For this review, take the finished solid that the model builds, in its own axes (mm). Face numbers are marked on the shaded views. A direction names the side the tool comes from. Give positions to 0.01 mm unless a question says otherwise; leave off trailing zeros. Write each loop counter-clockwise with the first axis right and the second up, starting at its lowest first coordinate (ties: lowest second). Pieces come first, ordered by that corner, then holes. Notation, with made-up numbers: M 17.25,-11.75 L 43.25,-11.75 A10 cw 43.25,-5.75 Z; hole C 64.5,-21.75 d8. An arc over 180 degrees is marked long. Use one line per item in the form item = value. Start each with the question number.
Q1. Clearance check with flat-ended pins moving along their axes: pin 1 Ø12 at (x, z) = (12, -5) entering from +Y; pin 2 Ø2 at (x, y) = (4, 32.5) entering from -Z; pin 3 Ø21.5 at (x, y) = (-8.5, 23) entering from +Z. State where each tip first meets the part, or that it passes through.
Q2. Consider section C-C on y = 21.5. Write out the cut boundary in (x, z), and give its area (3 significant figures).
Q3. Consider section D-D on z = -31. Write out the cut boundary in (x, y).
Q4. Consider section B-B on x = -15.5. Write out the cut boundary in (y, z).
Q5. Tool access review of the marked faces 1, 2 and 3: name each direction out of +Z, -Z, +X, -X, +Y, -Y from which nothing blocks a thin tool from reaching the whole face with its end or side.
Q6. For probe 1 along X at (y, z) = (-1, 31); probe 2 along Z at (x, y) = (-11, -1); probe 3 along Y at (x, z) = (11, 27), list the stretches that pass through material, from the lowest coordinate up. Write a range as [from, to].
Q7. Consider section A-A on y = 6. Write out the cut boundary in (x, z).
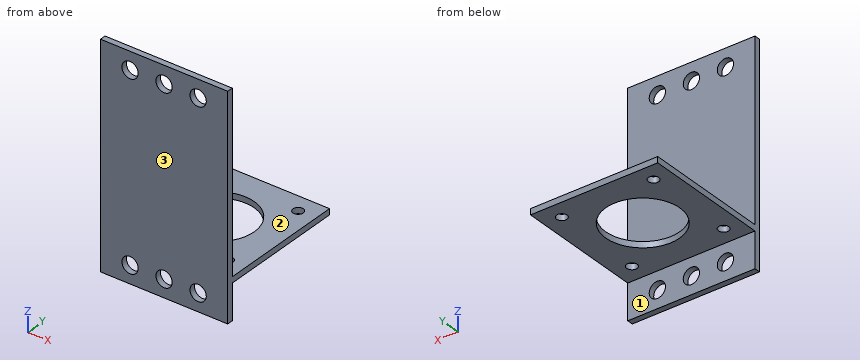
```python
from build123d import *

# Parameters (mm, degrees)
SKETCH1_W           = 43
SKETCH1_H           = 2
BOSS_EXTRUDE1_DEPTH = 43
SKETCH1_3_W         = 43
SKETCH1_3_H         = 74
BOSS_EXTRUDE2_DEPTH = 2
CUT_EXTRUDE1_REACH  = 78.885
SKETCH2_R           = 12.5
SKETCH2_R_2         = 1.75
CUT_EXTRUDE2_REACH  = 62.665
SKETCH1_4_R         = 2.75
LPATTERN1_COUNT     = 2
LPATTERN1_PITCH     = 11.5
LPATTERN1_COL_COUNT = 2
LPATTERN1_COL_PITCH = 11.5


with BuildPart() as part:
    # Sketch1 → Boss-Extrude1 (new body)
    with BuildSketch(Plane(origin=(0, 0, 0), x_dir=(1, 0, 0), z_dir=(0, 1, 0))):
        with Locations((0, 24)):
            Rectangle(SKETCH1_W, SKETCH1_H)
    extrude(amount=BOSS_EXTRUDE1_DEPTH)

    # Sketch1_3 → Boss-Extrude2 (add)
    with BuildSketch(Plane(origin=(0, 0, 0), x_dir=(1, 0, 0), z_dir=(0, 1, 0))):
        Rectangle(SKETCH1_3_W, SKETCH1_3_H)
    extrude(amount=-BOSS_EXTRUDE2_DEPTH)

    # Sketch2 → Cut-Extrude1 (cut, up to next)
    with BuildSketch(Plane.XY.offset(-23), mode=Mode.PRIVATE) as cut_extrude1_sk1:
        with Locations((0, 21.5)):
            Circle(SKETCH2_R)
    cut_extrude1_tool1 = extrude(cut_extrude1_sk1.sketch, amount=-CUT_EXTRUDE1_REACH, mode=Mode.PRIVATE) & part.part
    # Sketch2 → Cut-Extrude1 (cut, up to next)
    with BuildSketch(Plane.XY.offset(-23), mode=Mode.PRIVATE) as cut_extrude1_sk2:
        with Locations((-15.5, 37)):
            Circle(SKETCH2_R_2)
    cut_extrude1_tool2 = extrude(cut_extrude1_sk2.sketch, amount=-CUT_EXTRUDE1_REACH, mode=Mode.PRIVATE) & part.part
    # Sketch2 → Cut-Extrude1 (cut, up to next)
    with BuildSketch(Plane.XY.offset(-23), mode=Mode.PRIVATE) as cut_extrude1_sk3:
        with Locations((15.5, 37)):
            Circle(SKETCH2_R_2)
    cut_extrude1_tool3 = extrude(cut_extrude1_sk3.sketch, amount=-CUT_EXTRUDE1_REACH, mode=Mode.PRIVATE) & part.part
    # Sketch2 → Cut-Extrude1 (cut, up to next)
    with BuildSketch(Plane.XY.offset(-23), mode=Mode.PRIVATE) as cut_extrude1_sk4:
        with Locations((15.5, 6)):
            Circle(SKETCH2_R_2)
    cut_extrude1_tool4 = extrude(cut_extrude1_sk4.sketch, amount=-CUT_EXTRUDE1_REACH, mode=Mode.PRIVATE) & part.part
    # Sketch2 → Cut-Extrude1 (cut, up to next)
    with BuildSketch(Plane.XY.offset(-23), mode=Mode.PRIVATE) as cut_extrude1_sk5:
        with Locations((-15.5, 6)):
            Circle(SKETCH2_R_2)
    cut_extrude1_tool5 = extrude(cut_extrude1_sk5.sketch, amount=-CUT_EXTRUDE1_REACH, mode=Mode.PRIVATE) & part.part
    add(cut_extrude1_tool1.solids().sort_by_distance((0, 21.5, -23))[0], mode=Mode.SUBTRACT)
    add(cut_extrude1_tool2.solids().sort_by_distance((-15.5, 37, -23))[0], mode=Mode.SUBTRACT)
    add(cut_extrude1_tool3.solids().sort_by_distance((15.5, 37, -23))[0], mode=Mode.SUBTRACT)
    add(cut_extrude1_tool4.solids().sort_by_distance((15.5, 6, -23))[0], mode=Mode.SUBTRACT)
    add(cut_extrude1_tool5.solids().sort_by_distance((-15.5, 6, -23))[0], mode=Mode.SUBTRACT)

    # Sketch1_4 → Cut-Extrude2 (cut, up to next)
    with BuildSketch(Plane(origin=(0, 0, 0), x_dir=(1, 0, 0), z_dir=(0, 1, 0)), mode=Mode.PRIVATE) as cut_extrude2_sk1:
        with Locations(Location((0, 31, 0), (0, 0, 270))):
            Circle(SKETCH1_4_R)
    cut_extrude2_tool1 = extrude(cut_extrude2_sk1.sketch, amount=-CUT_EXTRUDE2_REACH, mode=Mode.PRIVATE) & part.part
    # Sketch1_4 → Cut-Extrude2 (cut, up to next)
    with BuildSketch(Plane(origin=(0, 0, 0), x_dir=(1, 0, 0), z_dir=(0, 1, 0)), mode=Mode.PRIVATE) as cut_extrude2_sk2:
        with Locations(Location((0, -31, 0), (0, 0, 270))):
            Circle(SKETCH1_4_R)
    cut_extrude2_tool2 = extrude(cut_extrude2_sk2.sketch, amount=-CUT_EXTRUDE2_REACH, mode=Mode.PRIVATE) & part.part
    cut_extrude2_1 = cut_extrude2_tool1.solids().sort_by_distance((0, 0, -31))[0]
    add(cut_extrude2_1, mode=Mode.SUBTRACT)
    cut_extrude2_2 = cut_extrude2_tool2.solids().sort_by_distance((0, 0, 31))[0]
    add(cut_extrude2_2, mode=Mode.SUBTRACT)
    cut_extrude2 = cut_extrude2_1 + cut_extrude2_2  # Cut-Extrude2 as one shape, for the pattern or mirror that repeats it

    # LPattern1: Cut-Extrude2 ×2
    with Locations(*[(i * LPATTERN1_PITCH, 0, 0) for i in range(1, LPATTERN1_COUNT)]):
        add(cut_extrude2, mode=Mode.SUBTRACT)

    # LPattern1 col: Cut-Extrude2 ×2
    with Locations(*[(-i * LPATTERN1_COL_PITCH, 0, 0) for i in range(1, LPATTERN1_COL_COUNT)]):
        add(cut_extrude2, mode=Mode.SUBTRACT)


solid = part.part
```
Working result:
q1.pin_1 = 0
q1.pin_2 = -25
q1.pin_3 = -23
q2.outline = M -21.5,-25 L -12.5,-25 L -12.5,-23 L -21.5,-23 Z; M 12.5,-25 L 21.5,-25 L 21.5,-23 L 12.5,-23 Z
q2.area = 36.0 mm²
q3.outline = M -21.5,-2 L -14.25,-2 L -14.25,0 L -21.5,0 Z; M -8.75,-2 L -2.75,-2 L -2.75,0 L -8.75,0 Z; M 2.75,-2 L 8.75,-2 L 8.75,0 L 2.75,0 Z; M 14.25,-2 L 21.5,-2 L 21.5,0 L 14.25,0 Z
q4.outline = M -2,-37 L 0,-37 L 0,-25 L 4.25,-25 L 4.25,-23 L 0,-23 L 0,37 L -2,37 Z; M 7.75,-25 L 35.25,-25 L 35.25,-23 L 7.75,-23 Z; M 38.75,-25 L 43,-25 L 43,-23 L 38.75,-23 Z
q5.face_1 = -Z, +X, -X, +Y
q5.face_2 = +Z, +X, -X, +Y
q5.face_3 = +Z, -Z, +X, -X, -Y
q6.probe_1 = [-21.5, -14.25], [-8.75, -2.75], [2.75, 8.75], [14.25, 21.5]
q6.probe_2 = [-37, -33.7], [-28.3, 28.3], [33.7, 37]
q6.probe_3 = [-2, 0]
q7.outline = M -21.5,-25 L -17.25,-25 L -17.25,-23 L -21.5,-23 Z; M -13.75,-25 L 13.75,-25 L 13.75,-23 L -13.75,-23 Z; M 17.25,-25 L 21.5,-25 L 21.5,-23 L 17.25,-23 Z
